Verification items for the finished model (mm, model axes). A direction names the side the tool comes from. Round coordinates to 2 decimals unless told otherwise and drop trailing zeros. Write each loop counter-clockwise with the first axis right and the second up, starting at its lowest first coordinate (ties: lowest second). Pieces come first, ordered by that corner, then holes. Notation, with made-up numbers: M 1,20.5 L 23,20.5 A22 ccw 23,36.5 Z; hole C 76,-33.75 d9. An arc over 180 degrees is marked long. Answer in a Markdown table with one row per item. Add a question column.
1. Go/stop test with flat-tipped pins: pin 1 Ø12.5 at (x, y) = (9, 7.5) entering from +Z; pin 2 Ø3.5 at (x, y) = (15.5, -15.5) entering from +Z. Record where each tip stops, or that it passes through.
2. Set-up check for faces 1 (the cylindrical face through (-0.54, -2.44, -23.88)), 2 (the flat face through (0, -21.15, -23)), 3 (the flat face through (9, -9, 0)): record each of +Z, -Z, +X, -X, +Y, -Y from which the full face is reachable in a straight line by a thin tool's end or side.
3. Sectioned sample at D-D on x = 0. Record the cut outline in (y, z), plus the area to 3 significant figures.
4. Sectioned sample at A-A on y = -15.5. Record the cut outline in (x, z).
5. Material ranges on probe 1 along Y at (x, z) = (0, -30); probe 2 along Y at (x, z) = (15.5, -26); probe 3 along X at (y, z) = (-14.5, -7.5), recorded low to high.
6. Sectioned sample at C-C on z = -23. Record the cut outline in (x, y).
7. Draft check along Y on faces 4 (the flat face through (-19, -18.9, -23.2)), 5 (the flat face through (0, 0, 0)), 6 (the flat face through (0, -4, -47.1)), 7 (the cylindrical face through (14, -15.43, -23.22)). Enter one of: pulls with the +Y half, pulls with the -Y half, needs draft (parallel to the pull), parting line crosses it, or undercut.
```python
from build123d import *

# Parameters (mm, degrees)
F0_R     = 1.5
F0_R_2   = 11.15
F0_R_3   = 2.5
F1_DEPTH = 47.1
F2_DEPTH = 2
F3_DEPTH = 24


with BuildPart() as f1:
    # F0 (on Top) → F1 (new body)
    with BuildSketch(Plane.XY):
        Polygon((-16.75, 21.15), (-21.15, 16.75), (-21.15, -16.75), (-16.75, -21.15), (16.75, -21.15), (21.15, -16.75), (21.15, 16.75), (16.75, 21.15), align=None)
        with Locations((-15.5, -15.5)):
            Circle(F0_R, mode=Mode.SUBTRACT)
        with Locations((15.5, -15.5)):
            Circle(F0_R, mode=Mode.SUBTRACT)
        with Locations((-15.5, 15.5)):
            Circle(F0_R, mode=Mode.SUBTRACT)
        Circle(F0_R_2, mode=Mode.SUBTRACT)
        with Locations((15.5, 15.5)):
            Circle(F0_R, mode=Mode.SUBTRACT)
        Circle(F0_R_2)
        Circle(F0_R_3, mode=Mode.SUBTRACT)
    extrude(amount=-F1_DEPTH)

    # F0 (on Top) → F2 (join)
    with BuildSketch(Plane.XY):
        Circle(F0_R_2)
        Circle(F0_R_3, mode=Mode.SUBTRACT)
    extrude(amount=F2_DEPTH)

    # F0 (on Top) → F3 (join)
    with BuildSketch(Plane.XY):
        Circle(F0_R_3)
    extrude(amount=F3_DEPTH)


solid = f1.part
```
Geometry check:
| question | item | result |
|---|---|---|
| 1 | pin 1 | stops at z = 2 |
| 1 | pin 2 | stops at z = 0 |
| 2 | face 1 | -Z |
| 2 | face 2 | +Z, -Z, +X, -X, -Y |
| 2 | face 3 | +Z |
| 3 | outline | M -21.15,-47.1 L -2.5,-47.1 L -2.5,0 L 2.5,0 L 2.5,-47.1 L 21.15,-47.1 L 21.15,0 L 11.15,0 L 11.15,2 L 2.5,2 L 2.5,24 L -2.5,24 L -2.5,2 L -11.15,2 L -11.15,0 L -21.15,0 Z |
| 3 | area | 1,910 mm2 |
| 4 | outline | M -21.15,-47.1 L -17,-47.1 L -17,0 L -21.15,0 Z; M -14,-47.1 L 14,-47.1 L 14,0 L -14,0 Z; M 17,-47.1 L 21.15,-47.1 L 21.15,0 L 17,0 Z |
| 5 | probe 1 | y = -21.15 to -2.5, 2.5 to 21.15 |
| 5 | probe 2 | y = -21.15 to -17, -14 to 14, 17 to 21.15 |
| 5 | probe 3 | x = -21.15 to -16.62, -14.38 to 14.38, 16.62 to 21.15 |
| 6 | outline | M -21.15,-16.75 L -16.75,-21.15 L 16.75,-21.15 L 21.15,-16.75 L 21.15,16.75 L 16.75,21.15 L -16.75,21.15 L -21.15,16.75 Z; hole C -15.5,-15.5 d3; hole C -15.5,15.5 d3; hole C 0,0 d5; hole C 15.5,-15.5 d3; hole C 15.5,15.5 d3 |
| 7 | face 4 | pulls with the -Y half |
| 7 | face 5 | undercut |
| 7 | face 6 | needs draft |
| 7 | face 7 | undercut |
